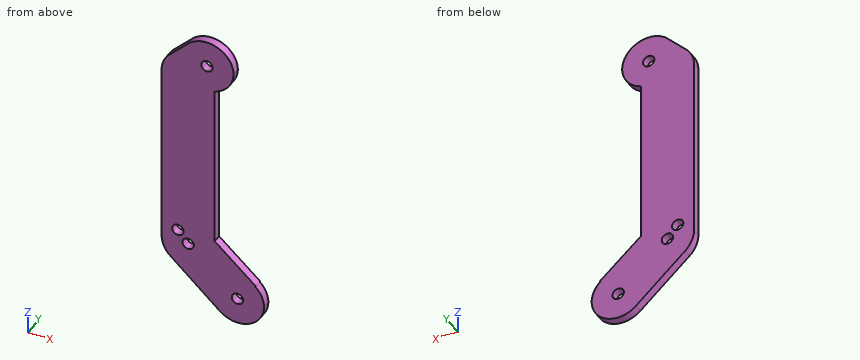
from build123d import *

# Parameters (mm, degrees)
F1_DEPTH = 3.2
F2_R     = 2.15
F3_DEPTH = 12.5


with BuildPart() as f1:
    # F0 (on Front) → F1 (new body)
    with BuildSketch(Plane.XZ):
        with BuildLine():
            Line((-18.5654132097, 100.885057482), (-25.6364810216, 93.8139896702))
            ThreePointArc((-25.6364810216, 93.8139896702), (-23.5654132097, 95.4031758961), (-21.1536036607, 96.4021801212))
            ThreePointArc((-21.1536036607, 96.4021801212), (-20.1545994357, 98.8139896702), (-18.5654132097, 100.885057482))
        make_face()
        with BuildLine():
            ThreePointArc((-6.6971687433, -7.4261652839), (-9.9867052636, -0.5154783973), (-7.4261652839, 6.6971687433))
            Line((-7.4261652839, 6.6971687433), (-11.1392479258, 10.045753115))
            ThreePointArc((-11.1392479258, 10.045753115), (-18.0499348124, 6.7562165947), (-25.262581953, 9.3167565744))
            Line((-25.262581953, 9.3167565744), (-6.6971687433, -7.4261652839))
        make_face()
        with BuildLine():
            Line((-28.5654132097, 86.7429218583), (-28.5654132097, 16.7429218583))
            ThreePointArc((-28.5654132097, 16.7429218583), (-25.6364810216, 23.8139896702), (-18.5654132097, 26.7429218583))
            Line((-18.5654132097, 26.7429218583), (-18.5654132097, 76.7429218583))
            ThreePointArc((-18.5654132097, 76.7429218583), (-25.6364810216, 79.6718540464), (-28.5654132097, 86.7429218583))
        make_face()
        with BuildLine():
            Line((-18.5654132097, 86.7429218583), (-28.5654132097, 86.7429218583))
            ThreePointArc((-28.5654132097, 86.7429218583), (-25.6364810216, 79.6718540464), (-18.5654132097, 76.7429218583))
            Line((-18.5654132097, 76.7429218583), (-18.5654132097, 86.7429218583))
        make_face()
        with BuildLine():
            ThreePointArc((-25.6364810216, 93.8139896702), (-27.8042085348, 90.5697561819), (-28.5654132097, 86.7429218583))
            Line((-28.5654132097, 86.7429218583), (-18.5654132097, 86.7429218583))
            ThreePointArc((-18.5654132097, 86.7429218583), (-21.1536036607, 91.2257992191), (-21.1536036607, 96.4021801212))
            ThreePointArc((-21.1536036607, 96.4021801212), (-23.5654132097, 95.4031758961), (-25.6364810216, 93.8139896702))
        make_face()
        with BuildLine():
            ThreePointArc((-8.9061549468, 84.1547314073), (-8.7353506369, 84.2021247154), (-8.5654132097, 84.2525380943))
            Line((-8.5654132097, 84.2525380943), (-8.5654132097, 86.7429218583))
            ThreePointArc((-8.5654132097, 86.7429218583), (-8.650964596, 85.4376599361), (-8.9061549468, 84.1547314073))
        make_face()
        with BuildLine():
            ThreePointArc((-11.8682444664, 24.1690871422), (-9.4283543987, 20.8066832051), (-8.5654132097, 16.7429218583))
            Line((-8.5654132097, 16.7429218583), (-8.5654132097, 21.2613671129))
            Line((-8.5654132097, 21.2613671129), (-11.8682444664, 24.1690871422))
        make_face()
        with BuildLine():
            ThreePointArc((-28.5654132097, 16.7429218583), (-27.7024720208, 12.6791605115), (-25.262581953, 9.3167565744))
            Line((-25.262581953, 9.3167565744), (-20.0053044895, 15.1462963223))
            ThreePointArc((-20.0053044895, 15.1462963223), (-20.5298808541, 15.8692131687), (-20.7154132097, 16.7429218583))
            Line((-20.7154132097, 16.7429218583), (-28.5654132097, 16.7429218583))
        make_face()
        with BuildLine():
            Line((6.6971687433, 7.4261652839), (1.4398912798, 1.596625536))
            ThreePointArc((1.4398912798, 1.596625536), (1.9644676444, 0.8737086896), (2.15, 0))
            ThreePointArc((2.15, 0), (0.8737086896, -1.9644676444), (-1.4398912798, -1.596625536))
            Line((-1.4398912798, -1.596625536), (-6.6971687433, -7.4261652839))
            ThreePointArc((-6.6971687433, -7.4261652839), (4.0637613468, -9.1370588111), (10, 0))
            ThreePointArc((10, 0), (9.1370588111, 4.0637613468), (6.6971687433, 7.4261652839))
        make_face()
        with BuildLine():
            Line((-7.4261652839, 6.6971687433), (-1.596625536, 1.4398912798))
            ThreePointArc((-1.596625536, 1.4398912798), (-0.1108278554, 2.1471416317), (1.4398912798, 1.596625536))
            Line((1.4398912798, 1.596625536), (6.6971687433, 7.4261652839))
            ThreePointArc((6.6971687433, 7.4261652839), (-0.5154783973, 9.9867052636), (-7.4261652839, 6.6971687433))
        make_face()
        with BuildLine():
            ThreePointArc((-1.4398912798, -1.596625536), (-2.1471416317, -0.1108278554), (-1.596625536, 1.4398912798))
            Line((-1.596625536, 1.4398912798), (-7.4261652839, 6.6971687433))
            ThreePointArc((-7.4261652839, 6.6971687433), (-9.9867052636, -0.5154783973), (-6.6971687433, -7.4261652839))
            Line((-6.6971687433, -7.4261652839), (-1.4398912798, -1.596625536))
        make_face()
        with BuildLine():
            Line((-11.1392479258, 10.045753115), (-7.4261652839, 6.6971687433))
            ThreePointArc((-7.4261652839, 6.6971687433), (-0.5154783973, 9.9867052636), (6.6971687433, 7.4261652839))
            Line((6.6971687433, 7.4261652839), (6.8974743638, 7.6482744619))
            Line((6.8974743638, 7.6482744619), (-8.5654132097, 21.2613671129))
            Line((-8.5654132097, 21.2613671129), (-8.5654132097, 16.7429218583))
            ThreePointArc((-8.5654132097, 16.7429218583), (-9.2310237589, 13.1555588183), (-11.1392479258, 10.045753115))
        make_face()
        with BuildLine():
            ThreePointArc((-25.262581953, 9.3167565744), (-18.0499348124, 6.7562165947), (-11.1392479258, 10.045753115))
            Line((-11.1392479258, 10.045753115), (-16.9687876737, 15.3030305785))
            ThreePointArc((-16.9687876737, 15.3030305785), (-18.4545853543, 14.5957802266), (-20.0053044895, 15.1462963223))
            Line((-20.0053044895, 15.1462963223), (-25.262581953, 9.3167565744))
        make_face()
        with BuildLine():
            ThreePointArc((-18.5654132097, 26.7429218583), (-25.6364810216, 23.8139896702), (-28.5654132097, 16.7429218583))
            Line((-28.5654132097, 16.7429218583), (-20.7154132097, 16.7429218583))
            ThreePointArc((-20.7154132097, 16.7429218583), (-20.0856927893, 18.2632014378), (-18.5654132097, 18.8929218583))
            Line((-18.5654132097, 18.8929218583), (-18.5654132097, 26.7429218583))
        make_face()
        with BuildLine():
            Line((-8.5654132097, 86.7429218583), (-8.5654132097, 84.2525380943))
            ThreePointArc((-8.5654132097, 84.2525380943), (-3.4541550431, 87.8679540951), (-1.4943453978, 93.8139896702))
            ThreePointArc((-1.4943453978, 93.8139896702), (-7.6675110742, 103.0527849953), (-18.5654132097, 100.885057482))
            ThreePointArc((-18.5654132097, 100.885057482), (-20.1545994357, 98.8139896702), (-21.1536036607, 96.4021801212))
            ThreePointArc((-21.1536036607, 96.4021801212), (-17.030591367, 96.624436009), (-13.1692451405, 95.1620293032))
            ThreePointArc((-13.1692451405, 95.1620293032), (-10.7796896928, 95.8417389701), (-9.3443453978, 93.8139896702))
            ThreePointArc((-9.3443453978, 93.8139896702), (-9.5551722221, 92.8854922849), (-10.1463057648, 92.1390899275))
            ThreePointArc((-10.1463057648, 92.1390899275), (-8.9687712332, 89.5544095029), (-8.5654132097, 86.7429218583))
        make_face()
        with BuildLine():
            Line((-11.8682444664, 24.1690871422), (-8.5654132097, 21.2613671129))
            Line((-8.5654132097, 21.2613671129), (-8.5654132097, 84.2525380943))
            ThreePointArc((-8.5654132097, 84.2525380943), (-8.7353506369, 84.2021247154), (-8.9061549468, 84.1547314073))
            ThreePointArc((-8.9061549468, 84.1547314073), (-12.4777989196, 78.8093884554), (-18.5654132097, 76.7429218583))
            Line((-18.5654132097, 76.7429218583), (-18.5654132097, 26.7429218583))
            ThreePointArc((-18.5654132097, 26.7429218583), (-14.9780501697, 26.0773113091), (-11.8682444664, 24.1690871422))
        make_face()
        with BuildLine():
            Line((-17.1255219299, 18.3395473943), (-11.8682444664, 24.1690871422))
            ThreePointArc((-11.8682444664, 24.1690871422), (-14.9780501697, 26.0773113091), (-18.5654132097, 26.7429218583))
            Line((-18.5654132097, 26.7429218583), (-18.5654132097, 18.8929218583))
            ThreePointArc((-18.5654132097, 18.8929218583), (-17.7941301561, 18.7498155902), (-17.1255219299, 18.3395473943))
        make_face()
        with BuildLine():
            Line((-16.4154132097, 16.7429218583), (-8.5654132097, 16.7429218583))
            ThreePointArc((-8.5654132097, 16.7429218583), (-9.4283543987, 20.8066832051), (-11.8682444664, 24.1690871422))
            Line((-11.8682444664, 24.1690871422), (-17.1255219299, 18.3395473943))
            ThreePointArc((-17.1255219299, 18.3395473943), (-16.6009455653, 17.6166305478), (-16.4154132097, 16.7429218583))
        make_face()
        with BuildLine():
            Line((-16.9687876737, 15.3030305785), (-11.1392479258, 10.045753115))
            ThreePointArc((-11.1392479258, 10.045753115), (-9.2310237589, 13.1555588183), (-8.5654132097, 16.7429218583))
            Line((-8.5654132097, 16.7429218583), (-16.4154132097, 16.7429218583))
            ThreePointArc((-16.4154132097, 16.7429218583), (-16.5585194778, 15.9716388047), (-16.9687876737, 15.3030305785))
        make_face()
        with BuildLine():
            ThreePointArc((-21.1536036607, 96.4021801212), (-21.1536036607, 91.2257992191), (-18.5654132097, 86.7429218583))
            Line((-18.5654132097, 86.7429218583), (-13.0146249774, 92.2937100906))
            ThreePointArc((-13.0146249774, 92.2937100906), (-13.6412283712, 93.6982593867), (-13.1692451405, 95.1620293032))
            ThreePointArc((-13.1692451405, 95.1620293032), (-17.030591367, 96.624436009), (-21.1536036607, 96.4021801212))
        make_face()
        with BuildLine():
            Line((-18.5654132097, 86.7429218583), (-8.5654132097, 86.7429218583))
            ThreePointArc((-8.5654132097, 86.7429218583), (-8.9687712332, 89.5544095029), (-10.1463057648, 92.1390899275))
            ThreePointArc((-10.1463057648, 92.1390899275), (-11.6100756813, 91.6671066968), (-13.0146249774, 92.2937100906))
            Line((-13.0146249774, 92.2937100906), (-18.5654132097, 86.7429218583))
        make_face()
        with BuildLine():
            ThreePointArc((-18.5654132097, 76.7429218583), (-12.4777989196, 78.8093884554), (-8.9061549468, 84.1547314073))
            ThreePointArc((-8.9061549468, 84.1547314073), (-14.0825358489, 84.1547314073), (-18.5654132097, 86.7429218583))
            Line((-18.5654132097, 86.7429218583), (-18.5654132097, 76.7429218583))
        make_face()
        with BuildLine():
            ThreePointArc((-8.9061549468, 84.1547314073), (-8.650964596, 85.4376599361), (-8.5654132097, 86.7429218583))
            Line((-8.5654132097, 86.7429218583), (-18.5654132097, 86.7429218583))
            ThreePointArc((-18.5654132097, 86.7429218583), (-14.0825358489, 84.1547314073), (-8.9061549468, 84.1547314073))
        make_face()
    extrude(amount=F1_DEPTH)

    # F2 (on Front) → F3 (cut, symmetric)
    with BuildSketch(Plane.XZ):
        with Locations((-22.4154132097, 21.2613671129)):
            Circle(F2_R)
    extrude(amount=F3_DEPTH, both=True, mode=Mode.SUBTRACT)


solid = f1.part
Geometry: final body of the model. Coordinates: model frame, mm. Give positions to 0.01 mm unless a question says otherwise; leave off trailing zeros. Write each loop counter-clockwise with the first axis right and the second up, starting at its lowest first coordinate (ties: lowest second). Pieces come first, ordered by that corner, then holes.
(1) First-contact query: P1, Ø1, axis at x = 4.5, y = -1.5, coming from the +Z side; P2, Ø1.5, axis at x = -2, y = -0.5, coming from the +Z side. Flat tips, straight axial feed; report the tip coordinate or a pass-through.
(2) Cut plane B-B, the plane x = -11.5. Return loops of the section in (y, z).
(3) Cut plane C-C, the plane x = 0. Return loops of the section in (y, z), then the cut area to 3 significant figures.
(4) Ray query, line 1 (X direction, y = -0.85, z = 37); line 2 (X direction, y = -2.7, z = 1); line 3 (X direction, y = -1.35, z = 23). Return the intervals inside material, ascending.
(5) Cut plane D-D, the plane z = 64. Return loops of the section in (x, y).
(6) Cut plane A-A, the plane y = -2.3. Return loops of the section in (x, z).
Values follow:
1. P1: stops at z = 10.2
1. P2: stops at z = 98.67
2. outline: (-3.2, -3.09) - (0, -3.09) - (0, 91.66) - (-3.2, 91.66) - close; (-3.2, 95.96) - (0, 95.96) - (0, 103.81) - (-3.2, 103.81) - close
3. outline: (-3.2, -10) - (0, -10) - (0, -2.15) - (-3.2, -2.15) - close; (-3.2, 2.15) - (0, 2.15) - (0, 13.72) - (-3.2, 13.72) - close
3. area: 62.1 mm2
4. line 1: x = -28.57 to -8.57
4. line 2: x = -16.04 to -1.9, 1.9 to 9.95
4. line 3: x = -28.57 to -23.68, -21.15 to -8.57
5. outline: (-28.57, -3.2) - (-8.57, -3.2) - (-8.57, 0) - (-28.57, 0) - close
6. outline: (-28.57, 16.74) arc R10 ccw to (-25.26, 9.32) - (-6.7, -7.43) arc R10 ccw to (6.7, 7.43) - (6.9, 7.65) - (-8.57, 21.26) - (-8.57, 84.25) arc R10 ccw (long way) to (-18.57, 100.89) - (-25.64, 93.81) arc R10 ccw to (-28.57, 86.74) - close; hole circle Ø4.3 at (-22.42, 21.26); hole circle Ø4.3 at (-18.57, 16.74); hole circle Ø4.3 at (-11.49, 93.81); hole circle Ø4.3 at (0, 0)
